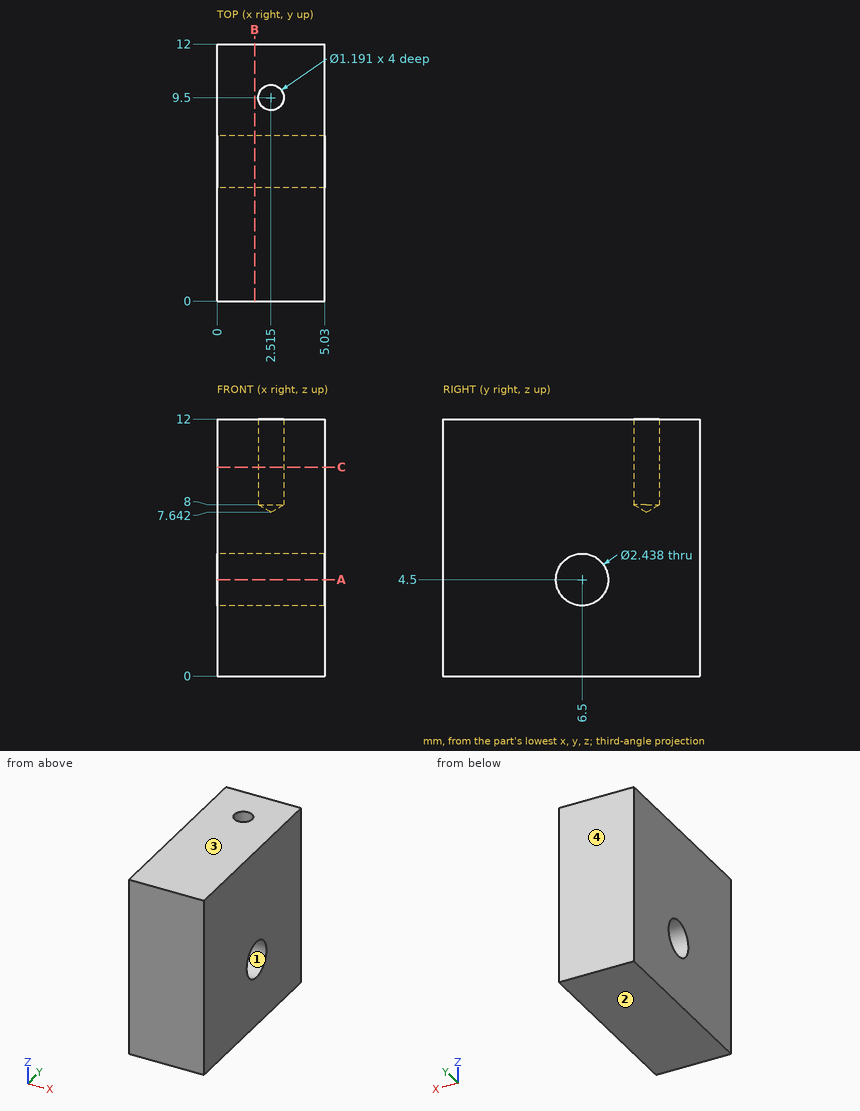
Verification items for this drawing (mm, ordinates from the low corner). Give positions to 0.01 mm unless a question says otherwise; leave off trailing zeros. Write each loop counter-clockwise with the first axis right and the second up, starting at its lowest first coordinate (ties: lowest second). Pieces come first, ordered by that corner, then holes. Notation, with made-up numbers: (49.25, 23.25) - (106.25, 23.25) arc R10 cw to (106.25, 37.25) - close; hole circle Ø10 at (26, 63). An arc over 180 degrees is marked (long way). Answer as CSV lines item,"result". Start each with the question number.
1. Sectioned sample at C-C (z = 9.75). Record the boundary of the cut face in (x, y) (1 decimal).
2. Depth check by flat-ended pin: pin 1 (2 mm diameter, centred on y = 8, z = 4, fed in from -X); pin 2 (2 mm diameter, centred on y = 6.5, z = 4.5, fed in from -X); pin 3 (1.1 mm diameter, centred on x = 2.515, y = 9.5, fed in from +Z). Enter the tip coordinate at first touch or a pass-through.
3. Thickness scan on line 1 (Y direction, x = 3, z = 4.5); line 2 (X direction, y = 9.5, z = 10.8); line 3 (Y direction, x = 2.55, z = 11.75) (1 decimal). Record the ranges inside material, lowest first.
4. Draft check along Z on the marked faces 1, 2, 3 and 4. Enter one of: pulls with the +Z half, pulls with the -Z half, needs draft (parallel to the pull), parting line crosses it, or undercut.
5. Sectioned sample at A-A (z = 4.5). Record the boundary of the cut face in (x, y).
6. Sectioned sample at B-B (x = 1.75). Record the boundary of the cut face in (y, z).
Derived:
1,outline,"(0, 0) - (5, 0) - (5, 12) - (0, 12) - close; hole circle Ø1.2 at (2.5, 9.5)"
2,pin 1,"x = 0"
2,pin 2,"through"
2,pin 3,"z = 7.97"
3,line 1,"0 to 5.28, 7.72 to 12"
3,line 2,"0 to 1.92, 3.11 to 5.03"
3,line 3,"0 to 8.9, 10.1 to 12"
4,face 1,"undercut"
4,face 2,"pulls with the -Z half"
4,face 3,"pulls with the +Z half"
4,face 4,"needs draft"
5,outline,"(0, 0) - (5.03, 0) - (5.03, 5.28) - (0, 5.28) - close; (0, 7.72) - (5.03, 7.72) - (5.03, 12) - (0, 12) - close"
6,outline,"(0, 0) - (12, 0) - (12, 12) - (0, 12) - close; hole circle Ø2.44 at (6.5, 4.5)"
